Here's the drawing with two shaded views (mm, measured from the low corner). I have some questions. A direction names the side the tool comes from. Give positions to 0.01 mm unless a question says otherwise; leave off trailing zeros. Order: outer loops, then holes, each group sorted by start corner. A loop starts at its lowest first (then second) coordinate and runs counter-clockwise, first axis right, second up. Notation, with made-up numbers: M 24.5,-14 L 45.5,-14 A29 ccw 45.5,25 Z; hole C 32.25,-5 d10. An arc over 180 degrees is marked long. Use a Markdown table: item, result. Add a question column.
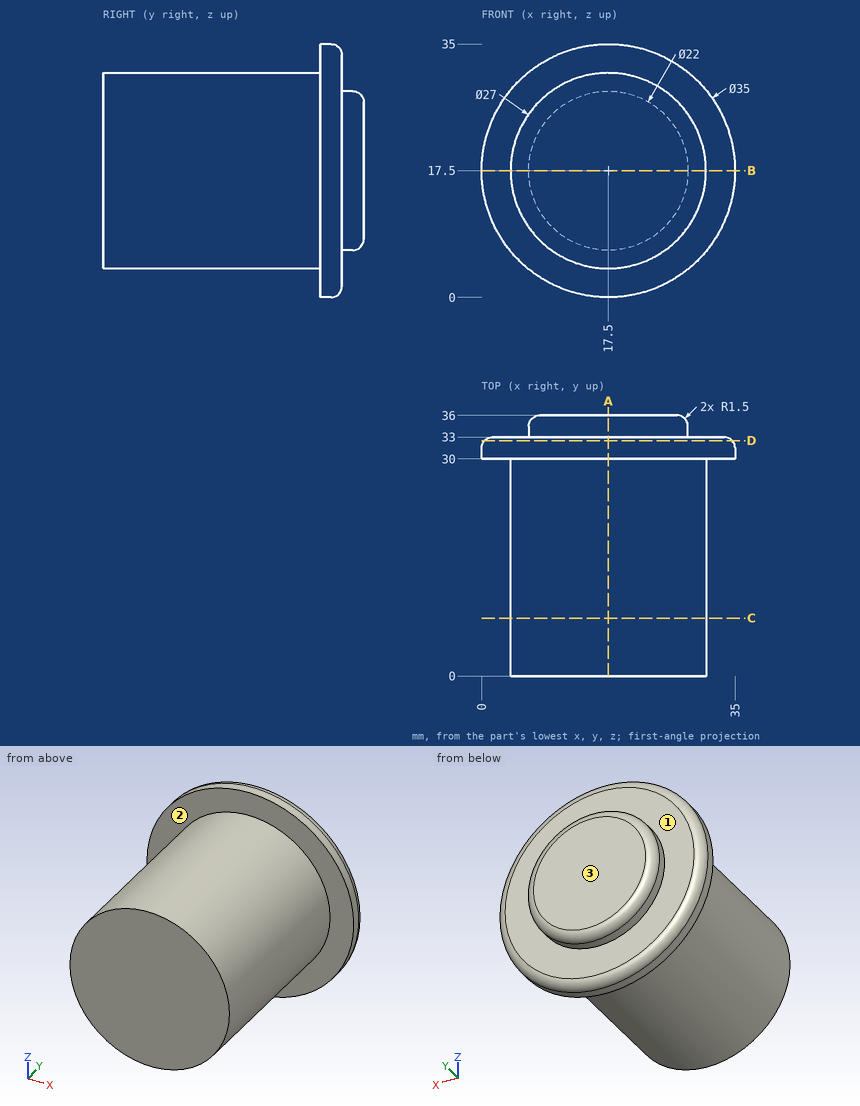
1) For pin 1 (4 mm diameter, centred on y = 25.5, z = 4, fed in from -X); pin 2 (6 mm diameter, centred on y = 12.5, z = 28, fed in from +X) (3 decimals); pin 3 (3 mm diameter, centred on x = 26, y = 12, fed in from +Z), each with a flat end and sliding along its axis, tell me the tip position at first contact or that it passes through.
2) Please list where these lines run through material, in increasing order: line 1 (Y direction, x = 10, z = 11.5); line 2 (Y direction, x = 5, z = 12.5); line 3 (Z direction, x = 9, y = 35). Write a range as from..to.
3) For the marked faces 1, 2 and 3, which set-ups out of +Z, -Z, +X, -X, +Y, -Y let a thin tool reach every point of the face, with its end or its side?
4) Suppose I cut it at D-D on y = 32.5. Please give me the cut outline in (x, z).
5) Suppose I cut it at A-A on x = 17.5. Please give me the cut outline in (y, z), and give its area (3 significant figures).
6) Suppose I cut it at C-C on y = 8. Please give me the cut outline in (x, z).
7) Suppose I cut it at B-B on z = 17.5. Please give me the cut outline in (x, y).
Values found:
| question | item | result |
|---|---|---|
| 1 | pin 1 | stops at x = 10.43 |
| 1 | pin 2 | stops at x = 28.725 |
| 1 | pin 3 | stops at z = 29.04 |
| 2 | line 1 | y = 0..36 |
| 2 | line 2 | y = 0..33 |
| 2 | line 3 | z = 10.65..24.35 |
| 3 | face 1 | +Y |
| 3 | face 2 | -Y |
| 3 | face 3 | +Z, -Z, +X, -X, +Y |
| 4 | outline | C 17.5,17.5 d34.24 |
| 5 | outline | M 0,4 L 30,4 L 30,0 L 31.5,0 A1.5 ccw 33,1.5 L 33,6.5 L 34.5,6.5 A1.5 ccw 36,8 L 36,27 A1.5 ccw 34.5,28.5 L 33,28.5 L 33,33.5 A1.5 ccw 31.5,35 L 30,35 L 30,31 L 0,31 Z |
| 5 | area | 979 mm^2 |
| 6 | outline | C 17.5,17.5 d27 |
| 7 | outline | M 0,30 L 4,30 L 4,0 L 31,0 L 31,30 L 35,30 L 35,31.5 A1.5 ccw 33.5,33 L 28.5,33 L 28.5,34.5 A1.5 ccw 27,36 L 8,36 A1.5 ccw 6.5,34.5 L 6.5,33 L 1.5,33 A1.5 ccw 0,31.5 Z |
